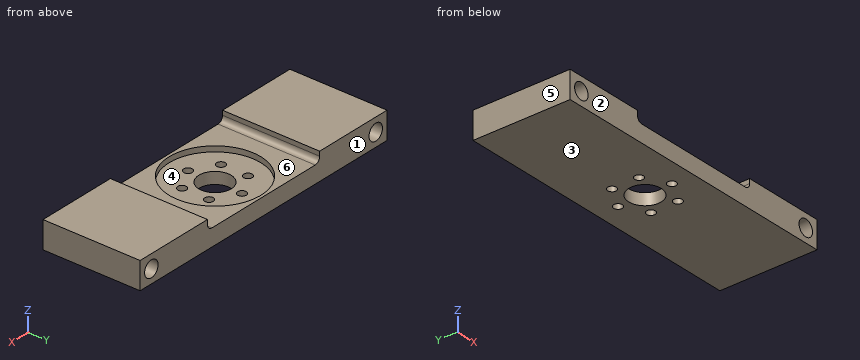
from build123d import *

# Parameters (mm, degrees)
BOSS_EXTRUDE1_DEPTH = 18
SKETCH9_R           = 8.5
CUT_EXTRUDE6_DEPTH  = 1
SKETCH10_R          = 3
CUT_EXTRUDE7_DEPTH  = 3.161013299
SKETCH11_R          = 0.8
CUT_EXTRUDE8_DEPTH  = 3.161013299
FILLET1_R           = 1
SKETCH13_R          = 1.5
CUT_EXTRUDE10_DEPTH = 19


with BuildPart() as part:
    # Sketch2 → Boss-Extrude1 (new body)
    with BuildSketch(Plane(origin=(0, 0, 0), x_dir=(1, 0, 0), z_dir=(0, 1, 0))):
        Polygon((-33.940224132, -1.838986701), (-18.940224132, -1.838986701), (-18.940224132, 3.161013299), (-73.940224132, 3.161013299), (-73.940224132, -1.838986701), (-58.940224132, -1.838986701), (-58.940224132, 0), (-33.940224132, 0), align=None)
    extrude(amount=BOSS_EXTRUDE1_DEPTH)

    # Sketch9 → Cut-Extrude6 (cut)
    with BuildSketch(Plane.XY):
        with Locations((-46.440224132, 9)):
            Circle(SKETCH9_R)
    extrude(amount=-CUT_EXTRUDE6_DEPTH, mode=Mode.SUBTRACT)

    # Sketch10 → Cut-Extrude7 (cut, through all)
    with BuildSketch(Plane.XY.offset(-1)):
        with Locations((-46.440224132, 9)):
            Circle(SKETCH10_R)
    extrude(amount=-CUT_EXTRUDE7_DEPTH, mode=Mode.SUBTRACT)

    # Sketch11 → Cut-Extrude8 (cut, through all)
    with BuildSketch(Plane.XY.offset(-1)):
        with Locations((-42.110097113, 11.5)):
            Circle(SKETCH11_R)
        with Locations((-42.110097113, 6.5)):
            Circle(SKETCH11_R)
        with Locations((-46.440224132, 14)):
            Circle(SKETCH11_R)
        with Locations((-46.440224132, 4)):
            Circle(SKETCH11_R)
        with Locations((-50.770351151, 11.5)):
            Circle(SKETCH11_R)
        with Locations((-50.770351151, 6.5)):
            Circle(SKETCH11_R)
    extrude(amount=-CUT_EXTRUDE8_DEPTH, mode=Mode.SUBTRACT)

    # Fillet1
    fillet1_edges = [part.edges().sort_by_distance(p)[0] for p in [
        (-33.940224132, 9, 0),
        (-58.940224132, 9, 0),
    ]]
    fillet(fillet1_edges, radius=FILLET1_R)

    # Sketch13 → Cut-Extrude10 (cut, through all)
    with BuildSketch(Plane(origin=(0, 18, 0), x_dir=(1, 0, 0), z_dir=(0, 1, 0))):
        with Locations((-71.440224132, 0.661013299)):
            Circle(SKETCH13_R)
        with Locations((-21.440224132, 0.661013299)):
            Circle(SKETCH13_R)
    extrude(amount=-CUT_EXTRUDE10_DEPTH, mode=Mode.SUBTRACT)


solid = part.part
Can you work these out from the model? Positions are in its coordinate system, mm. Face numbers are marked on the shaded views. A direction names the side the tool comes from. Round coordinates to 2 decimals unless told otherwise and drop trailing zeros. Loops run counter-clockwise (first coordinate to the right, second up) from the corner with the lowest first, then second, coordinate; pieces in that order, holes last. Notation, with made-up numbers: (51, 63.5) - (80, 63.5) arc R29 cw to (80, 93.5) - close; hole circle Ø8 at (33.5, 31). An arc over 180 degrees is marked (long way). Answer in a Markdown table with one row per item. Add a question column.
Q1. I want a section at D-D on x = -48. List the corners of the cut face in (y, z) for me, and give its area (3 significant figures).
Q2. We'd pull the mould along Y, two halves only. Please class the marked faces 1, 2, 3 and 4: pulls with the +Y half, pulls with the -Y half, needs draft (parallel to the pull), parting line crosses it, or undercut.
Q3. I want a section at A-A on y = 9. List the corners of the cut face in (x, z) for me, and give its area (3 significant figures).
Q4. I want a section at B-B on z = -1.65. Count the separate pieces of the cut face and the enclosed holes in it, and give its area (3 significant figures).
Q5. Which directions (+Z, -Z, +X, -X, +Y, -Y) give clear straight access to the entire face, cutting with the end or side of a thin tool? Please do the marked faces 5 and 6.
Q6. I want a section at C-C on y = 6.5. List the corners of the cut face in (x, z) for me, and give its area (3 significant figures).
Q7. For pin 1 Ø5.5 at (x, y) = (-48, 6.5) entering from +Z; pin 2 Ø2.5 at (x, z) = (-21.44, -0.66) entering from -Y, each with a flat end and sliding along its axis, tell me the tip position at first contact or that it passes through.
Q8. I need wall thicknesses on L1, parallel to X at y = 14.5, z = -0.7; L2, parallel to X at y = 8.75, z = -2.3; L3, parallel to X at y = 7.75, z = -0.1. Which ranges of each line are inside material? Lowest first, please.
A:
| question | item | result |
|---|---|---|
| 1 | outline | (0, -3.16) - (6.44, -3.16) - (6.44, -1) - (0.64, -1) - (0.64, 0) - (0, 0) - close; (11.56, -3.16) - (18, -3.16) - (18, 0) - (17.36, 0) - (17.36, -1) - (11.56, -1) - close |
| 1 | area | 29.1 mm^2 |
| 2 | face 1 | pulls with the +Y half |
| 2 | face 2 | pulls with the -Y half |
| 2 | face 3 | needs draft |
| 2 | face 4 | undercut |
| 3 | outline | (-73.94, -3.16) - (-49.44, -3.16) - (-49.44, -1) - (-54.94, -1) - (-54.94, 0) - (-57.94, 0) arc R1 cw to (-58.94, 1) - (-58.94, 1.84) - (-73.94, 1.84) - close; (-43.44, -3.16) - (-18.94, -3.16) - (-18.94, 1.84) - (-33.94, 1.84) - (-33.94, 1) arc R1 cw to (-34.94, 0) - (-37.94, 0) - (-37.94, -1) - (-43.44, -1) - close; hole circle Ø3 at (-71.44, -0.66); hole circle Ø3 at (-21.44, -0.66) |
| 3 | area | 185 mm^2 |
| 4 | separate pieces | 3 |
| 4 | enclosed holes | 7 |
| 4 | area | 868 mm^2 |
| 5 | face 5 | +Z, -Z, -X, +Y, -Y |
| 5 | face 6 | +Z, +Y, -Y |
| 6 | outline | (-73.94, -3.16) - (-51.57, -3.16) - (-51.57, -1) - (-54.56, -1) - (-54.56, 0) - (-57.94, 0) arc R1 cw to (-58.94, 1) - (-58.94, 1.84) - (-73.94, 1.84) - close; (-49.97, -3.16) - (-48.1, -3.16) - (-48.1, -1) - (-49.97, -1) - close; (-44.78, -3.16) - (-42.91, -3.16) - (-42.91, -1) - (-44.78, -1) - close; (-41.31, -3.16) - (-18.94, -3.16) - (-18.94, 1.84) - (-33.94, 1.84) - (-33.94, 1) arc R1 cw to (-34.94, 0) - (-38.32, 0) - (-38.32, -1) - (-41.31, -1) - close; hole circle Ø3 at (-71.44, -0.66); hole circle Ø3 at (-21.44, -0.66) |
| 6 | area | 185 mm^2 |
| 7 | pin 1 | z = -1 |
| 7 | pin 2 | through |
| 8 | L1 | -73.94 to -72.94, -69.94 to -52.92, -39.96 to -22.94, -19.94 to -18.94 |
| 8 | L2 | -73.94 to -49.43, -43.45 to -18.94 |
| 8 | L3 | -73.94 to -72.83, -70.05 to -54.85, -38.03 to -22.83, -20.05 to -18.94 |
